```python
from build123d import *

# Parameters (mm, degrees)
SKETCH6_R                  = 1
BOSS_EXTRUDE1_DEPTH        = 2
CUT_EXTRUDE1_DEPTH         = 72.147733625
CUT_EXTRUDE1_DEPTH_BACK    = 72.147733625
M10X1_0_TAPPED_HOLE1_D     = 9
M10X1_0_TAPPED_HOLE1_DEPTH = 9
M10X1_0_TAPPED_HOLE1_TIP   = 2.703872786
CHAMFER1_SIZE              = 2
CHAMFER1_SIZE2             = 1
CHAMFER2_SIZE2             = 0.5
CHAMFER2_SIZE              = 1.37373871


with BuildPart() as part:
    # Sketch1 → Revolve1 (revolve)
    with BuildSketch(Plane.XY, mode=Mode.PRIVATE) as revolve1_sk:
        Polygon((7.5, 0), (7.5, -46), (9, -46), (9, -47.5), (7.5, -47.5), (7.5, -56.5), (7, -56.5), (7, -70), (3.35, -70), (3.35, 0), align=None)
    revolve(revolve1_sk.sketch.rotate(Axis((0, -80.784886464, 0), (0, 1, 0)), 90), axis=Axis((0, -80.784886464, 0), (0, 1, 0)))

    # Sketch6 → Boss-Extrude1 (add)
    with BuildSketch(Plane(origin=(0, 0, 0), x_dir=(1, 0, 0), z_dir=(0, 1, 0))):
        with Locations(Location((6.499, 0, 0), (0, 0, 270))):
            Circle(SKETCH6_R)
    extrude(amount=BOSS_EXTRUDE1_DEPTH)

    # Sketch2 → Cut-Revolve1 (revolve, cut)
    with BuildSketch(Plane.XY, mode=Mode.PRIVATE) as cut_revolve1_sk:
        Polygon((-3.35, 0), (-4.25, 0), (-4.25, -30), (-4, -30), (-4, -40), (-3.35, -40), align=None)
    revolve(cut_revolve1_sk.sketch.rotate(Axis((0, -73.381951652, 0), (0, 1, 0)), 270), axis=Axis((0, -73.381951652, 0), (0, 1, 0)), mode=Mode.SUBTRACT)

    # Sketch3 → Cut-Extrude1 (cut, two sides: drawn at the far end of the back side and taken through both)
    with BuildSketch(Plane(origin=(0, 0, 0), x_dir=(0, 0, -1), z_dir=(1, 0, 0)).offset(-CUT_EXTRUDE1_DEPTH_BACK)):
        with BuildLine():
            Line((-1.55, -27.95), (-1.55, -14.05))
            ThreePointArc((-1.55, -14.05), (0, -12.5), (1.55, -14.05))
            Line((1.55, -14.05), (1.55, -27.95))
            ThreePointArc((1.55, -27.95), (0, -29.5), (-1.55, -27.95))
        make_face()
    extrude(amount=CUT_EXTRUDE1_DEPTH + CUT_EXTRUDE1_DEPTH_BACK, mode=Mode.SUBTRACT)

    # M10x1.0 Tapped Hole1
    with Locations(Plane(origin=(0, 0, 0), x_dir=(-1, 0, 0), z_dir=(0, 1, 0))):
        with Locations((0, 0)):
            Hole(M10X1_0_TAPPED_HOLE1_D / 2, depth=M10X1_0_TAPPED_HOLE1_DEPTH)
            with Locations((0, 0, -(M10X1_0_TAPPED_HOLE1_DEPTH + M10X1_0_TAPPED_HOLE1_TIP / 2))):  # 118° drill point
                Cone(0, M10X1_0_TAPPED_HOLE1_D / 2, M10X1_0_TAPPED_HOLE1_TIP, mode=Mode.SUBTRACT)

    # Chamfer1
    chamfer1_edges = [part.edges().sort_by_distance(p)[0] for p in [
        (0, -70, 7),
    ]]
    chamfer1_side = [part.faces().sort_by_distance(p)[0] for p in [
        (0, -63.25, 7),
    ]]
    chamfer(chamfer1_edges, length=CHAMFER1_SIZE, length2=CHAMFER1_SIZE2, reference=chamfer1_side[0])

    # Chamfer2
    chamfer2_edges = [part.edges().sort_by_distance(p)[0] for p in [
        (0, -56.5, 7),
    ]]
    chamfer2_side = [part.faces().sort_by_distance(p)[0] for p in [
        (0, -56.51, 7),
    ]]
    chamfer(chamfer2_edges, length=CHAMFER2_SIZE - 0.0001, length2=CHAMFER2_SIZE2 - 0.0001, reference=chamfer2_side[0])  # a hair under: the kernel refuses the full size


solid = part.part
```
Here's how the part is built. I have some questions about the finished solid (model axes, mm). A direction names the side the tool comes from. Coordinates: 2 decimals unless noted, no trailing zeros. Loops run counter-clockwise (first coordinate to the right, second up) from the corner with the lowest first, then second, coordinate; pieces in that order, holes last. Notation, with made-up numbers: (24.5, -5) - (45.5, -5) arc R9 cw to (45.5, 11) - close; hole circle Ø3 at (-16.75, -28). An arc over 180 degrees is marked (long way). Return JSON: item names as keys, results as strings. Group by question number.
Item 1: Will these pins go through, and if not, where does the flat tip stop? P1, Ø1.7, axis at x = 5, y = -23.5, coming from the +Z side; P2, Ø2.5, axis at x = 5.5, y = -21.5, coming from the -Z side; P3, Ø1, axis at x = -5, y = -39, coming from the +Z side; P4, Ø4, axis at x = 0, z = 1, coming from the +Y side.
Item 2: If we section it at A-A on y = -19: Write out the boundary of the cut face in (x, z), and give its area (3 significant figures).
Item 3: On a 3-axis mill with a long thin cutter (end or side, diameter ignored), from which of +Z, -Z, +X, -X, +Y, -Y can I reach the whole of each face in a straight line? I mean faces 1 (the face through (-7.4, -46, -2)), 2 (the face through (-6.083, -46.76, 6.633)), 3 (the face through (-5.8, -29.5, 0)). Say none if no direction works.
Item 4: If we section it at C-C on y = -51.5: Write out the boundary of the cut face in (x, z), and give its area (3 significant figures).
Item 5: If we section it at B-B on z = 0: State how many separate pieces and enclosed holes the cut face has, and give its area (3 significant figures).
Item 6: I need wall thicknesses on line 1 (X direction, y = -9, z = 0); line 2 (X direction, y = -35.5, z = 0); line 3 (Y direction, x = 8.25, z = 1). Which ranges of each line are inside material? Lowest first, please. Write a range as from..to.
Item 7: We'd pull the mould along Y, two halves only. Please class faces 4 (the face through (6, -21, 1.55)), 5 (the face through (-3.4, 0, 3.2)), 6 (the face through (6.5, 1, -1)): +Y half, -Y half, draft (parallel to the pull), parting line (faces both ways), or undercut.
Calculated:
{
 "1": {"P1": "stops at z = 6.25", "P2": "stops at z = -6.18", "P3": "stops at z = 6", "P4": "passes through"},
 "2": {"outline": "(-7.34, -1.55) arc R7.5 ccw to (7.34, -1.55) - (3.96, -1.55) arc R4.25 cw to (-3.96, -1.55) - close; (-7.34, 1.55) - (-3.96, 1.55) arc R4.25 cw to (3.96, 1.55) - (7.34, 1.55) arc R7.5 ccw to start", "area": "99.6 mm^2"},
 "3": {"face 1": "+Y", "face 2": "+Y, -Y", "face 3": "+X, -X"},
 "4": {"outline": "circle Ø15 at (0, 0); hole circle Ø6.7 at (0, 0)", "area": "141 mm^2"},
 "5": {"separate pieces": "4", "enclosed holes": "0", "area": "393 mm^2"},
 "6": {"line 1": "x = -7.5..-4.5, 4.5..7.5", "line 2": "x = -7.5..-4, 4..7.5", "line 3": "y = -47.5..-46"},
 "7": {"face 4": "undercut", "face 5": "+Y half", "face 6": "draft"}
}
